Part model, mm, in its own coordinate system. A direction names the side the tool comes from. Round coordinates to 2 decimals unless told otherwise and drop trailing zeros. Loops run counter-clockwise (first coordinate to the right, second up) from the corner with the lowest first, then second, coordinate; pieces in that order, holes last. Notation, with made-up numbers: M 0.25,74 L 51.25,74 A23 cw 51.25,101 Z; hole C -26,-16 d9. An arc over 180 degrees is marked long. Write each question's results on one line, items separated by ' | '.
from build123d import *

# Parameters (mm, degrees)
SKETCH1_W           = 12.7
SKETCH1_H           = 12.7
BOSS_EXTRUDE1_DEPTH = 2.54
FILLET1_R           = 0.635
SHELL1_START        = 0.635
SHELL1_OUTLINE_W    = 1.905
SHELL1_OUTLINE_H    = 11.43
SHELL1_DEPTH        = 11.43
SKETCH2_R           = 2.54
BOSS_EXTRUDE2_DEPTH = 1.905
BOSS_EXTRUDE3_DEPTH = 0.00254


# Read off the part's stored shape, not the designer's step: Shell1
with BuildPart() as part:
    # Sketch1 → Boss-Extrude1 (new body)
    with BuildSketch(Plane(origin=(0, 0, 0), x_dir=(1, 0, 0), z_dir=(0, 1, 0))):
        with Locations((6.35, 6.35)):
            Rectangle(SKETCH1_W, SKETCH1_H)
    extrude(amount=BOSS_EXTRUDE1_DEPTH)

    # Fillet1
    fillet1_edges = [part.edges().sort_by_distance(p)[0] for p in [
        (0, 1.27, -12.7),
        (12.7, 1.27, -12.7),
        (12.7, 1.27, 0),
        (0, 1.27, 0),
    ]]
    fillet(fillet1_edges, radius=FILLET1_R)

    # Shell1 outline → Shell1 (cut)
    with BuildSketch(Plane.YZ.offset(SHELL1_START)):
        with Locations((0.9525, -6.35)):
            Rectangle(SHELL1_OUTLINE_W, SHELL1_OUTLINE_H)
    extrude(amount=SHELL1_DEPTH, mode=Mode.SUBTRACT)

    # Sketch2 → Boss-Extrude2 (add)
    with BuildSketch(Plane(origin=(0, 1.905, 0), x_dir=(-1, 0, 0), z_dir=(0, -1, 0))):
        with Locations(Location((-6.35, 6.35, 0), (0, 0, 270))):
            Circle(SKETCH2_R)
    extrude(amount=BOSS_EXTRUDE2_DEPTH)

    # Sketch3 → Boss-Extrude3 (add)
    with BuildSketch(Plane(origin=(0, 2.54, 0), x_dir=(1, 0, 0), z_dir=(0, 1, 0))):
        with BuildLine():
            Line((7.771926803, 7.496002003), (7.340706851, 7.083226562))
            add(Edge.make_bspline(
                [(7.340706851, 7.083226562), (7.306566415, 7.117407905), (7.239577243, 7.184477342), (7.130024832, 7.271772823), (7.016561783, 7.345991239), (6.898814643, 7.407018813), (6.776619389, 7.454357105), (6.650217166, 7.4882197), (6.519402332, 7.508304178), (6.430846529, 7.511115937), (6.386044391, 7.512538462)],
                knots=[0, 0, 0, 0, 1.075575784, 2.110457258, 3.113929901, 4.09197124, 5.059417775, 6.02750972, 7.002078037, 8, 8, 8, 8], degree=3))
            add(Edge.make_bspline(
                [(6.386044391, 7.512538462), (6.347202307, 7.511541705), (6.270932472, 7.509584486), (6.158861293, 7.494721502), (6.051770417, 7.469893554), (5.949153902, 7.435498578), (5.851638258, 7.390739844), (5.758658459, 7.33630815), (5.670786706, 7.271787088), (5.588714925, 7.198399755), (5.513988304, 7.118275604), (5.448748017, 7.03251443), (5.39317731, 6.942714749), (5.347431283, 6.848417132), (5.312623532, 6.749766307), (5.287775353, 6.64683389), (5.272002938, 6.539919017), (5.270140687, 6.466980583), (5.269197436, 6.430036458)],
                knots=[0, 0, 0, 0, 1.075001177, 2.110859044, 3.123021556, 4.114053297, 5.101481495, 6.087880186, 7.091499647, 8.114004866, 9.131394192, 10.11971144, 11.092043119, 12.050101265, 13.015322563, 13.981809771, 14.977764287, 16, 16, 16, 16], degree=3))
            add(Edge.make_bspline(
                [(5.269197436, 6.430036458), (5.270077255, 6.391813648), (5.271810619, 6.316509478), (5.288461543, 6.205997372), (5.314115158, 6.099676762), (5.35166521, 5.998336523), (5.397877952, 5.900588436), (5.456483323, 5.808325972), (5.52482305, 5.720140184), (5.602775019, 5.637566437), (5.687566632, 5.561453315), (5.779398707, 5.495796177), (5.87547715, 5.439148239), (5.977352671, 5.394284903), (6.083257013, 5.358264559), (6.19426435, 5.332867125), (6.31012472, 5.317285888), (6.389175206, 5.31541236), (6.42929359, 5.314461538)],
                knots=[0, 0, 0, 0, 1.022067601, 2.013613092, 2.983553406, 3.943623673, 4.90013463, 5.87121881, 6.861774014, 7.881098904, 8.905697761, 9.905387765, 10.89678721, 11.884561068, 12.87834324, 13.885584958, 14.926927371, 16, 16, 16, 16], degree=3))
            add(Edge.make_bspline(
                [(6.42929359, 5.314461538), (6.455389112, 5.314696994), (6.50662043, 5.315159245), (6.581768042, 5.322662884), (6.653741405, 5.333390208), (6.722819251, 5.347591911), (6.78830408, 5.367689869), (6.851102574, 5.391191957), (6.910846789, 5.418929106), (6.967212798, 5.4518583), (7.021039491, 5.488767902), (7.07182304, 5.531000335), (7.120454247, 5.577603414), (7.166364864, 5.629146461), (7.20877784, 5.686090332), (7.249051978, 5.747388607), (7.286726148, 5.813649634), (7.308986821, 5.860439815), (7.320354287, 5.884333333)],
                knots=[0, 0, 0, 0, 1.109579412, 2.178351274, 3.208885622, 4.204702371, 5.174744997, 6.119429583, 7.05542196, 7.97267548, 8.893247984, 9.828544973, 10.778894627, 11.756245826, 12.760884819, 13.796418446, 14.874735809, 16, 16, 16, 16], degree=3))
            Line((7.320354287, 5.884333333), (6.408941026, 5.884333333))
            Line((6.408941026, 5.884333333), (6.408941026, 6.454205128))
            Line((6.408941026, 6.454205128), (7.991988902, 6.454205128))
            Line((7.991988902, 6.454205128), (7.996441026, 6.318733373))
            add(Edge.make_bspline(
                [(7.996441026, 6.318733373), (7.995868961, 6.283940789), (7.994725852, 6.214417712), (7.984279039, 6.110909693), (7.966974052, 6.008774494), (7.943316479, 5.908114696), (7.913667554, 5.808436526), (7.875855895, 5.710694487), (7.831578672, 5.614225725), (7.781969186, 5.519440156), (7.726222397, 5.428490826), (7.666202793, 5.342373816), (7.602765995, 5.261238176), (7.534532278, 5.18621433), (7.462564154, 5.116672044), (7.386719952, 5.052878855), (7.306731416, 4.994780786), (7.223022277, 4.941887042), (7.13511573, 4.895528796), (7.043495085, 4.855203272), (6.948298678, 4.820955656), (6.849280734, 4.792880061), (6.746636094, 4.771217506), (6.64036256, 4.756363463), (6.530401766, 4.746269974), (6.455817686, 4.745156592), (6.417845272, 4.744589744)],
                knots=[0, 0, 0, 0, 1.006889344, 2.011981806, 3.007738725, 4.003571281, 5.003404394, 6.015442001, 7.03424805, 8.074616296, 9.110249922, 10.119753985, 11.111721717, 12.089233633, 13.052717867, 14.006597561, 14.955430184, 15.912305663, 16.870361111, 17.829300583, 18.807640451, 19.796414044, 20.806216501, 21.841577364, 22.90109906, 24, 24, 24, 24], degree=3))
            add(Edge.make_bspline(
                [(6.417845272, 4.744589744), (6.377331282, 4.745149516), (6.297020469, 4.746259153), (6.178270169, 4.756651657), (6.062964889, 4.773803815), (5.951075868, 4.797541814), (5.842343325, 4.827085651), (5.736954077, 4.864170155), (5.635123675, 4.908283344), (5.536547184, 4.958257086), (5.442484518, 5.014931662), (5.353146488, 5.077313277), (5.269020717, 5.145803203), (5.189245497, 5.219254905), (5.115684686, 5.299473831), (5.045596958, 5.383859699), (4.982377825, 5.475507443), (4.923309052, 5.571445818), (4.870831882, 5.671634621), (4.824939843, 5.774220808), (4.785803137, 5.878610404), (4.754942899, 5.985289482), (4.729887276, 6.093514186), (4.711959507, 6.203755162), (4.701834859, 6.315998608), (4.70016576, 6.391432018), (4.699325641, 6.429400441)],
                knots=[0, 0, 0, 0, 1.084149091, 2.14910686, 3.187506334, 4.202448172, 5.208724393, 6.201130722, 7.189831603, 8.176984443, 9.156919086, 10.126598231, 11.090766514, 12.05840148, 13.026036446, 14.001772938, 14.991905635, 16.003017641, 17.015720547, 18.016462227, 19.009322657, 19.99686681, 20.986544154, 21.980959929, 22.983742515, 24, 24, 24, 24], degree=3))
            add(Edge.make_bspline(
                [(4.699325641, 6.429400441), (4.70045074, 6.481197483), (4.702672477, 6.583481286), (4.72324913, 6.734145976), (4.755325067, 6.87989903), (4.801357267, 7.020209626), (4.860427449, 7.155271043), (4.931698831, 7.285400345), (5.016719582, 7.410459214), (5.082531483, 7.487888023), (5.115917187, 7.527166867)],
                knots=[0, 0, 0, 0, 1.034044851, 2.041932006, 3.031217818, 4.011390712, 4.986069675, 5.97149666, 6.970960976, 8, 8, 8, 8], degree=3))
            add(Edge.make_bspline(
                [(5.115917187, 7.527166867), (5.136646046, 7.549890869), (5.177792517, 7.59499767), (5.243565077, 7.657674489), (5.311005647, 7.716593018), (5.381048291, 7.770503925), (5.453324806, 7.820587348), (5.528043218, 7.865904431), (5.604811571, 7.907898096), (5.684228565, 7.944423986), (5.765878441, 7.977172494), (5.850122815, 8.004882336), (5.936330711, 8.02942667), (6.025265506, 8.048098613), (6.116028744, 8.063647182), (6.209264693, 8.074068647), (6.304719281, 8.081706839), (6.369279964, 8.082173929), (6.401944832, 8.082410256)],
                knots=[0, 0, 0, 0, 1.020590567, 2.025856924, 3.013483481, 3.991664875, 4.957826714, 5.930500614, 6.890802512, 7.860442893, 8.829981142, 9.809047939, 10.802672283, 11.803273349, 12.823572789, 13.857849586, 14.916166035, 16, 16, 16, 16], degree=3))
            add(Edge.make_bspline(
                [(6.401944832, 8.082410256), (6.436090224, 8.081883676), (6.504027016, 8.080835974), (6.605037776, 8.073586558), (6.704644924, 8.062402419), (6.802428705, 8.045625571), (6.898717283, 8.024936226), (6.993012244, 7.998428055), (7.085928747, 7.968309997), (7.146417038, 7.944297656), (7.176614303, 7.932310096)],
                knots=[0, 0, 0, 0, 1.03180557, 2.052914215, 3.058998889, 4.059601663, 5.049854447, 6.033765722, 7.018406786, 8, 8, 8, 8], degree=3))
            add(Edge.make_bspline(
                [(7.176614303, 7.932310096), (7.202021565, 7.921231433), (7.253699235, 7.898697739), (7.328883874, 7.857471289), (7.40425221, 7.811767038), (7.47899098, 7.759913932), (7.552986303, 7.70200896), (7.62701077, 7.638966722), (7.70030871, 7.570052109), (7.747744937, 7.521005039), (7.771926803, 7.496002003)],
                knots=[0, 0, 0, 0, 0.894392155, 1.819168899, 2.76525314, 3.739198753, 4.75366411, 5.797420238, 6.877176959, 8, 8, 8, 8], degree=3))
        make_face()
    extrude(amount=BOSS_EXTRUDE3_DEPTH)


solid = part.part
Item 1: Band-saw the part on C-C on x = 9.5. Give the cut face in (y, z) (3 decimals).
Filled sheet:
outline: M 0,-12.7 L 2.54,-12.7 L 2.54,0 L 0,0 L 0,-0.635 L 1.905,-0.635 L 1.905,-12.065 L 0,-12.065 Z
Item 2: Drop a flat-ended pin along its axis: P1, Ø3, axis at x = 5, z = -11, coming from the +Y side. Give the stop position or say it passes through.
Filled sheet:
P1: y = 2.54
Item 3: Wall check: L1, parallel to X at y = 0.25, z = -12 (3 decimals); L2, parallel to Z at x = 12, y = 1.35 (3 decimals); L3, parallel to Z at x = 7, y = 0.9 (3 decimals). Give the ranges that are in metal, low to high.
Filled sheet:
L1: 0 to 0.635, 12.065 to 12.7 | L2: -12.7 to -12.065, -0.635 to 0 | L3: -12.7 to -12.065, -8.805 to -3.895, -0.635 to 0
Item 4: Band-saw the part on B-B on z = -2.25. Give the cut face in (x, y) (3 decimals), and give its area (3 significant figures).
Filled sheet:
outline: M 0,0 L 0.635,0 L 0.635,1.905 L 12.065,1.905 L 12.065,0 L 12.7,0 L 12.7,2.54 L 0,2.54 Z | area: 10.5 mm^2
Item 5: Band-saw the part on A-A on y = 0.8. Give the cut face in (x, z) (3 decimals).
Filled sheet:
outline: M 0,-12.065 A0.635 ccw 0.635,-12.7 L 12.065,-12.7 A0.635 ccw 12.7,-12.065 L 12.7,-0.635 A0.635 ccw 12.065,0 L 0.635,0 A0.635 ccw 0,-0.635 Z; C 6.35,-6.35 d5.08; hole M 0.635,-12.065 L 12.065,-12.065 L 12.065,-0.635 L 0.635,-0.635 Z
Item 6: Two-plate mould, pull along Z, no slides. Class faces 1 (the flat face through (12.065, 1, -6)), 2 (the flat face through (0, 1, -6)), 3 (the flat face through (6, 1, 0)), 4 (the flat face through (6, 1, -12.7)): +Z half, -Z half, draft (parallel to the pull), parting line (faces both ways), or undercut.
Filled sheet:
face 1: undercut | face 2: draft | face 3: +Z half | face 4: -Z half
Item 7: Which spindle directions (+Z, -Z, +X, -X, +Y, -Y) get a long thin tool onto all of the face, cutting with end or side? Do faces 5 (the flat face through (5.8, 0, -0.3)), 6 (the flat face through (5, 1.905, -9)). Say none if no direction does.
Filled sheet:
face 5: +Z, -Z, +X, -X, -Y | face 6: -Y
